Check sheet for the modelled part. Datum: model origin and axes. Units: mm. Round coordinates to 2 decimals unless told otherwise and drop trailing zeros. Write each loop counter-clockwise with the first axis right and the second up, starting at its lowest first coordinate (ties: lowest second). Pieces come first, ordered by that corner, then holes. Notation, with made-up numbers: M -19.75,-2 L -0.75,-2 A20 ccw -0.75,16 Z; hole C -15,61 d10. An arc over 180 degrees is marked long. One line per item, written item: value.
from build123d import *

# Parameters (mm, degrees)
SKETCH1_R           = 7.14375
SKETCH1_R_2         = 3.175
BOSS_EXTRUDE1_DEPTH = 2.38125
BOSS_EXTRUDE2_START = 1.5875
SKETCH2_R           = 7.540625
SKETCH2_R_2         = 3.175
BOSS_EXTRUDE2_DEPTH = 1.5875
SKETCH3_R           = 7.540625
SKETCH3_R_2         = 3.175
BOSS_EXTRUDE3_DEPTH = 1.5875


with BuildPart() as part:
    # Sketch1 → Boss-Extrude1 (new body)
    with BuildSketch(Plane.XY):
        with Locations(Location((0, 0, 0), (0, 0, 180))):
            Circle(SKETCH1_R)
        with Locations(Location((0, 0, 0), (0, 0, 180))):
            Circle(SKETCH1_R_2, mode=Mode.SUBTRACT)
    extrude(amount=BOSS_EXTRUDE1_DEPTH)

    # Sketch2 → Boss-Extrude2 (add)
    with BuildSketch(Plane(origin=(0, 0, 0), x_dir=(-1, 0, 0), z_dir=(0, 0, -1)).offset(BOSS_EXTRUDE2_START)):
        Circle(SKETCH2_R)
        Circle(SKETCH2_R_2, mode=Mode.SUBTRACT)
    extrude(amount=-BOSS_EXTRUDE2_DEPTH)

    # Sketch3 → Boss-Extrude3 (add)
    with BuildSketch(Plane.XY.offset(2.38125)):
        with Locations(Location((0, 0, 0), (0, 0, 180))):
            Circle(SKETCH3_R)
        with Locations(Location((0, 0, 0), (0, 0, 180))):
            Circle(SKETCH3_R_2, mode=Mode.SUBTRACT)
    extrude(amount=BOSS_EXTRUDE3_DEPTH)


solid = part.part
Q1. Scan lines: line 1 (Z direction, x = -5, y = -5.5); line 2 (Y direction, x = 0, z = -0.65) (3 decimals); line 3 (Y direction, x = 0, z = 1.5) (3 decimals). Record each from-to range of solid material in increasing order. Write a range as [from, to].
Completed:
line 1: [-1.59, 0], [2.38, 3.97]
line 2: [-7.541, -3.175], [3.175, 7.541]
line 3: [-7.144, -3.175], [3.175, 7.144]
Q2. Sectioned sample at D-D on x = 5. Enter the section's corners in (y, z), and give its area (3 significant figures).
Completed:
outline: M -5.64,-1.59 L 5.64,-1.59 L 5.64,0 L 5.1,0 L 5.1,2.38 L 5.64,2.38 L 5.64,3.97 L -5.64,3.97 L -5.64,2.38 L -5.1,2.38 L -5.1,0 L -5.64,0 Z
area: 60.1 mm^2
Q3. Draft check along Z on faces 1 (the cylindrical face through (7.137, -0.314, 1.174)), 2 (the cylindrical face through (7.533, -0.332, 3.164)), 3 (the flat face through (-3, -2, -1.588)). Enter one of: pulls with the +Z half, pulls with the -Z half, needs draft (parallel to the pull), parting line crosses it, or undercut.
Completed:
face 1: undercut
face 2: needs draft
face 3: pulls with the -Z half
Q4. Depth check by flat-ended pin: P1, Ø7.5, axis at x = 0, y = 0, coming from the -Z side; P2, Ø1, axis at x = 2.5, z = 1, coming from the -Y side; P3, Ø1.5, axis at y = 1, z = 1, coming from the +X side; P4, Ø3, axis at y = 1.5, z = 1, coming from the -X side. Enter the tip coordinate at first touch or a pass-through.
Completed:
P1: z = -1.59
P2: y = -6.86
P3: x = 7.14
P4: x = -7.53
